Work out the finished part from the listing and answer in its coordinate system (mm). Face numbers are marked on the shaded views. A direction names the side the tool comes from. Coordinates: 2 decimals unless noted, no trailing zeros. Order: outer loops, then holes, each group sorted by start corner. A loop starts at its lowest first (then second) coordinate and runs counter-clockwise, first axis right, second up. Notation, with made-up numbers: (86.5, 76.5) - (94.5, 76.5) arc R13 cw to (94.5, 98.5) - close; hole circle Ø1 at (-37.75, -14.75). An arc over 180 degrees is marked (long way). Answer as a JSON object with one key per item and string values. Group by question number.
1) Section C-C (z = -6) is taken. Give the vertices of the cut face in (x, y), plus the area to 3 significant figures.
2) Find the intervals of material crossed by line 1 along Z through (x, y) = (0, -6.75); line 2 along X through (y, z) = (-33, -8); line 3 along Y through (x, z) = (-4, -3), in increasing order.
3) Section A-A (x = 0) is taken. Give the vertices of the cut face in (y, z), plus the area to 3 significant figures.
4) A tool of negligible diameter and unlimited length cuts with its end or side. For the marked faces 1, 2, 3, 4 and 5, from which of +Z, -Z, +X, -X, +Y, -Y can it reach the whole face along a straight path? Write none if from no direction.
5) Section B-B (y = -39.5) is taken. Give the vertices of the cut face in (x, z), plus the area to 3 significant figures.
6) The mould has two halves that part along Y. Classify the marked faces 6, 7 and 8: released by +Y, released by -Y, zero draft, split by the parting line, or undercut.
7) Each of these flat-tipped pins is pushed along its axis until it touches: P1, Ø5, axis at x = 8.5, y = -15.5, coming from the +Z side; P2, Ø5, axis at x = -11.5, y = -16, coming from the -Z side; P3, Ø1.5, axis at x = 5.5, y = -39.5, coming from the +Z side. Where does it stop, or does it pass through?
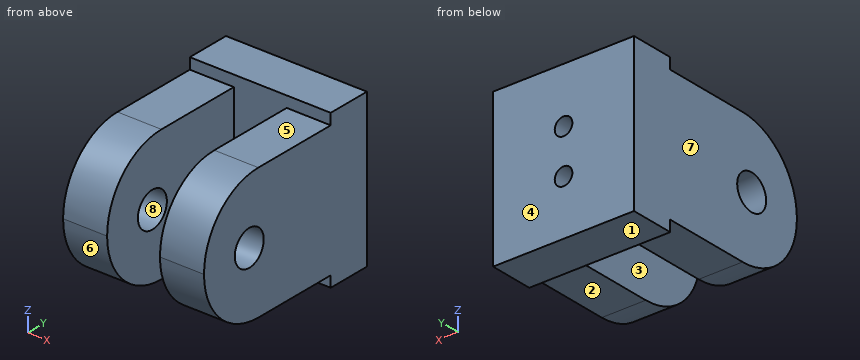
from build123d import *

# Parameters (mm, degrees)
F0_W      = 32
F0_H      = 35
F1_DEPTH  = 10
F2_W      = 10
F2_H      = 30
F3_DEPTH  = 35
F4_R      = 4
F5_DEPTH  = 10.001
F6_R      = 4
F7_DEPTH  = 10.001
F8_R      = 14.99999
F9_R      = 2
F10_DEPTH = 10.001


# Not quite as in the source:
# - a fillet or chamfer is up to 0.001 mm smaller than in the source, because OpenCascade refuses the exact size


with BuildPart() as f1:
    # F0 (on Front) → F1 (new body)
    with BuildSketch(Plane.XZ):
        Rectangle(F0_W, F0_H)
    extrude(amount=F1_DEPTH)

    # F2 (on face) → F3 (join)
    with BuildSketch(Plane.XZ.offset(10)):
        with Locations((-11, 0)):
            Rectangle(F2_W, F2_H)
        with Locations((11, 0)):
            Rectangle(F2_W, F2_H)
    extrude(amount=F3_DEPTH)

    # F4 (on face) → F5 (cut, through all)
    with BuildSketch(Plane.YZ.offset(-6)):
        with Locations((-32.5, 0)):
            Circle(F4_R)
    extrude(amount=-F5_DEPTH, mode=Mode.SUBTRACT)

    # F6 (on face) → F7 (cut, through all)
    with BuildSketch(Plane(origin=(6, 0, 0), x_dir=(0, -1, 0), z_dir=(-1, 0, 0))):
        with Locations((32.5, 0)):
            Circle(F6_R)
    extrude(amount=-F7_DEPTH, mode=Mode.SUBTRACT)

    # F8 (radius 15 in the source; OpenCascade refuses exactly that, so slightly less here)
    f8_edges = [f1.edges().sort_by_distance(p)[0] for p in [
        (-11, -45, -15),
        (11, -45, -15),
        (-11, -45, 15),
        (11, -45, 15),
    ]]
    fillet(f8_edges, radius=F8_R)

    # F9 (on face) → F10 (cut, through all)
    with BuildSketch(Plane.XZ.offset(10)):
        with Locations((0, 5)):
            Circle(F9_R)
        with Locations((0, -5)):
            Circle(F9_R)
    extrude(amount=-F10_DEPTH, mode=Mode.SUBTRACT)


solid = f1.part
Report:
{
 "1": {"outline": "(-16, -43.75) - (-6, -43.75) - (-6, -10) - (-1.73, -10) - (-1.73, 0) - (-16, 0) - close; (1.73, -10) - (6, -10) - (6, -43.75) - (16, -43.75) - (16, 0) - (1.73, 0) - close", "area": "960 mm²"},
 "2": {"line 1": "z = -17.5 to -7, -3 to 3, 7 to 17.5", "line 2": "x = -16 to -6, 6 to 16", "line 3": "y = -10 to 0"},
 "3": {"outline": "(-10, -17.5) - (0, -17.5) - (0, -7) - (-10, -7) - close; (-10, -3) - (0, -3) - (0, 3) - (-10, 3) - close; (-10, 7) - (0, 7) - (0, 17.5) - (-10, 17.5) - close", "area": "270 mm²"},
 "4": {"face 1": "-Z, +X, -X, +Y, -Y", "face 2": "-Z, +X, -X, -Y", "face 3": "+Z, -Z, -Y", "face 4": "+Z, -Z, +X, -X, +Y", "face 5": "+Z, +X, -X, -Y"},
 "5": {"outline": "(-16, -11.61) - (-6, -11.61) - (-6, 11.61) - (-16, 11.61) - close; (6, -11.61) - (16, -11.61) - (16, 11.61) - (6, 11.61) - close", "area": "464 mm²"},
 "6": {"face 6": "released by -Y", "face 7": "zero draft", "face 8": "undercut"},
 "7": {"P1": "stops at z = 15", "P2": "stops at z = -15", "P3": "stops at z = 12.04"}
}
